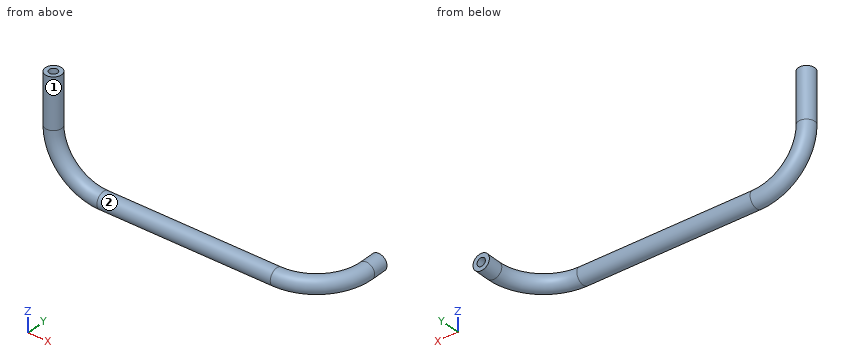
```python
from build123d import *

# Parameters (mm, degrees)
F0_R   = 12.5
F0_R_2 = 6.35


with BuildPart() as f4:
    # F4: sweep along a path in F1, F3
    with BuildLine(Plane.XY) as f4_path:
        Line((0, 0), (0, -23.8))
        ThreePointArc((0, -23.8), (-22.3184632736, -77.6815367264), (-76.2, -100))
        Line((-76.2, -100), (-340.5, -100))
    with BuildLine(Plane.XZ.offset(100)) as f4_path_2:
        ThreePointArc((-340.5, 0), (-394.3815367264, 22.3184632736), (-416.7, 76.2))
        Line((-416.7, 76.2), (-416.7, 153.261))
    # F0 (on Front) → F4 (sweep)
    with BuildSketch(Plane.XZ):
        Circle(F0_R)
        Circle(F0_R_2, mode=Mode.SUBTRACT)
    sweep(path=f4_path.line + f4_path_2.line)


solid = f4.part
```
Could you check a few things on this model? Use its own coordinates, in mm. Face numbers are marked on the shaded views. Round coordinates to 2 decimals unless told otherwise and drop trailing zeros. Loops run counter-clockwise (first coordinate to the right, second up) from the corner with the lowest first, then second, coordinate; pieces in that order, holes last. Notation, with made-up numbers: (45, 32) - (102, 32) arc R31 cw to (102, 58) - close; hole circle Ø1 at (-22, 51.25). An arc over 180 degrees is marked (long way). Answer in a Markdown table with one row per item. Add a question column.
(1) If we section it at A-A (x = -329): Please give me the cut outline in (y, z), plus the area to 3 significant figures.
(2) If we section it at B-B (z = 124.5): Please give me the cut outline in (x, y), plus the area to 3 significant figures.
(3) I'm going to push flat-ended pins straight in: pin 1 (16.5 mm diameter, centred on y = -100, z = 0, fed in from +X); pin 2 (1 mm diameter, centred on x = -123.5, y = -86.5, fed in from -Z); pin 3 (7.5 mm diameter, centred on x = 0, z = 0, fed in from -Y); pin 4 (6 mm diameter, centred on y = -96, z = 116.5, fed in from +X). Where does each tip first touch, or does it pass through?
(4) If we mould it in two halves opening along X, with no side actions, what happens to the marked faces 1 and 2? For each: pulls with the +X half, pulls with the -X half, needs draft (parallel to the pull), parting line crosses it, or undercut.
(5) I need wall thicknesses on line 1 along Z through (x, y) = (-245, -100); line 2 along Y through (x, z) = (-134.5, 0); line 3 along X through (y, z) = (-100, 133). Which ranges of each line are inside material? Lowest first, please.
Model answer:
| question | item | result |
|---|---|---|
| 1 | outline | circle Ø25 at (-100, 0); hole circle Ø12.7 at (-100, 0) |
| 1 | area | 364 mm² |
| 2 | outline | circle Ø25 at (-416.7, -100); hole circle Ø12.7 at (-416.7, -100) |
| 2 | area | 364 mm² |
| 3 | pin 1 | stops at x = -19.19 |
| 3 | pin 2 | passes through |
| 3 | pin 3 | stops at y = -74.97 |
| 3 | pin 4 | stops at x = -404.24 |
| 4 | face 1 | parting line crosses it |
| 4 | face 2 | undercut |
| 5 | line 1 | z = -12.5 to -6.35, 6.35 to 12.5 |
| 5 | line 2 | y = -112.5 to -106.35, -93.65 to -87.5 |
| 5 | line 3 | x = -429.2 to -423.05, -410.35 to -404.2 |
